Geometry check sheet. Reference: the model listing, model coordinates, mm. Face numbers are marked on the shaded views. A direction names the side the tool comes from. Coordinates: 2 decimals unless noted, no trailing zeros. Loops run counter-clockwise (first coordinate to the right, second up) from the corner with the lowest first, then second, coordinate; pieces in that order, holes last. Notation, with made-up numbers: M -4,40 L 6,40 A16 cw 6,66 Z; hole C -33,-36.75 d8. An arc over 180 degrees is marked long. One line per question, with ' | ' between items. Start each with the question number.
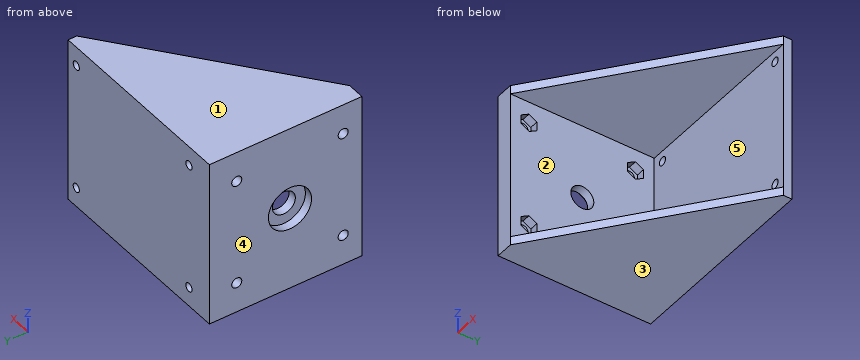
Autodesk Inventor part; units mm, degrees
ref_plane "YZ Plane" through (0, 0, 0) normal (1, 0, 0) x (0, 1, 0)
ref_plane "XZ Plane" through (0, 0, 0) normal (0, 1, 0) x (-1, 0, 0)
ref_plane "XY Plane" through (0, 0, 0) normal (0, 0, 1) x (1, 0, 0)
sketch "Skizze1" plane through (0, 0, 0) normal (0, 1, 0) x (-1, 0, 0)
  line L0 (-31.5, -26) -> (31.5, -26)
  line L1 (31.5, -26) -> (31.5, 26)
  line L2 (31.5, 26) -> (-31.5, 26)
  line L3 (-31.5, 26) -> (-31.5, -26)
  line L4 (-31.5, -26) -> (31.5, 26) construction
  line L5 (31.5, -26) -> (-31.5, 26) construction
  circle A0 centre (27.5, 22.25) radius 1.5
  circle A1 centre (-27.5, 22.25) radius 1.5
  circle A2 centre (-27.5, -22.25) radius 1.5
  circle A3 centre (27.5, -22.25) radius 1.5
  line L6 (31.5, 0) -> (-31.5, 0) construction
  line L7 (0, 26) -> (0, -26) construction
  line L8 (31.5, -26) -> (31.5, 26)
  line L9 (31.5, 26) -> (37.5, 26)
  line L10 (37.5, 26) -> (37.5, -26)
  line L11 (37.5, -26) -> (31.5, -26)
  point P0 (0, 0)
  dimension "d0" = 63
  dimension "d1" = 52
  dimension "d4" = 3
  dimension "d9" = 44.5
  dimension "d10" = 55
  dimension "d11" = 6
extrude "Extrusion1" add sketch "Skizze1" along normal blind 3
extrude "Extrusion2" add sketch "Skizze1" against normal blind 50 contours L1 L9 L10 L11
sketch "Skizze2" plane through (-31.5, -50, 26) normal (1, 0, 0) x (0, 0, -1)
  line L0 (52, 0) -> (0, 0)
  line L1 (26, 50) -> (26, 0) construction
  line L2 (7.5, 6.5) -> (44.5, 6.5)
  line L3 (44.5, 6.5) -> (44.5, 43.5)
  line L4 (44.5, 43.5) -> (7.5, 43.5)
  line L5 (7.5, 43.5) -> (7.5, 6.5)
  line L6 (7.5, 6.5) -> (44.5, 43.5) construction
  line L7 (44.5, 6.5) -> (7.5, 43.5) construction
  line L8 (42.9123, 3.75) -> (41.3246, 6.5)
  line L9 (41.3246, 6.5) -> (42.9123, 9.25)
  line L10 (42.9123, 9.25) -> (46.0877, 9.25)
  line L11 (46.0877, 9.25) -> (47.6754, 6.5)
  line L12 (47.6754, 6.5) -> (46.0877, 3.75)
  line L13 (46.0877, 3.75) -> (42.9123, 3.75)
  line L14 (5.9123, 3.75) -> (4.3246, 6.5)
  line L15 (4.3246, 6.5) -> (5.9123, 9.25)
  line L16 (5.9123, 9.25) -> (9.0877, 9.25)
  line L17 (9.0877, 9.25) -> (10.6754, 6.5)
  line L18 (10.6754, 6.5) -> (9.0877, 3.75)
  line L19 (9.0877, 3.75) -> (5.9123, 3.75)
  line L20 (41.3246, 43.5) -> (42.9123, 46.25)
  line L21 (42.9123, 46.25) -> (46.0877, 46.25)
  line L22 (46.0877, 46.25) -> (47.6754, 43.5)
  line L23 (47.6754, 43.5) -> (46.0877, 40.75)
  line L24 (46.0877, 40.75) -> (42.9123, 40.75)
  line L25 (42.9123, 40.75) -> (41.3246, 43.5)
  line L26 (4.3246, 43.5) -> (5.9123, 46.25)
  line L27 (5.9123, 46.25) -> (9.0877, 46.25)
  line L28 (9.0877, 46.25) -> (10.6754, 43.5)
  line L29 (10.6754, 43.5) -> (9.0877, 40.75)
  line L30 (9.0877, 40.75) -> (5.9123, 40.75)
  line L31 (5.9123, 40.75) -> (4.3246, 43.5)
  circle A0 centre (44.5, 6.5) radius 1.75
  circle A1 centre (7.5, 6.5) radius 1.75
  circle A2 centre (44.5, 43.5) radius 1.75
  circle A3 centre (7.5, 43.5) radius 1.75
  circle A4 centre (26, 25) radius 4
  point P0 (26, 25)
  dimension "d30" = 37
  dimension "d31" = 37
  dimension "d39" = 5.5
  dimension "d42" = 3.5
  dimension "d45" = 8
extrude "Extrusion4" cut sketch "Skizze2" against normal through all contours L5 A1 L2 | L2 A1 L5 | A0 L3 L2 | L2 L3 A0 | A3 L4 L5 | L5 L4 A3 | A2 L4 L3 | L3 L4 A2 | A4
extrude "Extrusion3" cut sketch "Skizze2" against normal blind 3 contours L5 A1 L2 | L2 A1 L5 | A1 L5 L16 L17 L2 | L2 L18 L19 L14 L15 L16 L5 A1 | L9 L10 L3 A0 L2 | L2 A0 L3 L10 L11 L12 L13 L8 | L30 L31 L26 L27 L28 L4 A3 L5 | L5 A3 L4 L29 L30 | A0 L3 L2 | L2 L3 A0 | A3 L4 L5 | L5 L4 A3 | L24 L25 L4 A2 L3 | L3 A2 L4 L20 L21 L22 L23 L24 | A2 L4 L3 | L3 L4 A2
sketch "Skizze3" plane through (31.5, 3, -26) normal (0, 0, -1) x (-1, 0, 0)
  line L0 (0, -3) -> (63, -3)
  line L1 (63, -3) -> (63, -53)
  line L2 (69, -53) -> (63, -53)
  line L3 (69, -53) -> (69, 0)
  line L4 (0, 0) -> (69, 0)
  line L5 (0, -3) -> (0, 0)
  line L6 (63, -53) -> (0, -3)
  point P0 (31.5, -3)
extrude "Extrusion5" add sketch "Skizze3" along normal blind 3
sketch "Skizze4" plane through (-37.5, 3, 26) normal (0, 0, 1) x (1, 0, 0)
  line L0 (6, -3) -> (69, -3)
  line L1 (69, -3) -> (69, 0)
  line L2 (0, 0) -> (69, 0)
  line L3 (0, -53) -> (0, 0)
  line L4 (6, -53) -> (0, -53)
  line L5 (6, -3) -> (6, -53)
  line L6 (6, -53) -> (69, -3)
  point P0 (37.5, -3)
extrude "Extrusion6" add sketch "Skizze4" along normal blind 3
sketch "Skizze5" plane through (-37.5, -50, -29) normal (-1, 0, 0) x (0, 0, 1)
  circle A0 centre (29, 25) radius 4
  circle A1 centre (29, 25) radius 7.5
  point P0 (29, 50)
  dimension "d51" = 15
extrude "Extrusion7" cut sketch "Skizze5" against normal blind 3
equation "\"d31\" = d30"
properties part number "Sanftanlauf_Halter"
1. Sectioned sample at B-B (y = -25). Record the cut outline in (x, z).
2. Sectioned sample at D-D (y = -36.5). Record the cut outline in (x, z).
3. Sectioned sample at C-C (z = 0). Record the cut outline in (x, y), and give its area (3 significant figures).
4. Tool access check on the marked faces 4 and 5. Record the directions out of +Z, -Z, +X, -X, +Y, -Y that give a thin tool (end or side, any length) a straight path to the whole face; none if there is none.
5. Depth check by flat-ended pin: pin 1 Ø10 at (x, y) = (-17, -41.5) entering from -Z; pin 2 Ø8 at (y, z) = (-38.5, 0.5) entering from +X; pin 3 Ø3 at (x, z) = (6, -17) entering from -Y. Enter the tip coordinate at first touch or a pass-through.
6. Thickness scan on line 1 (Y direction, x = -35.2, z = -18.5); line 2 (Z direction, x = -27.5, y = 1.3); line 3 (Z direction, x = -27, y = -7). Record the ranges inside material, lowest first.
7. Draft check along Z on the marked faces 1, 2 and 3. Enter one of: +Z half, -Z half, draft (parallel to the pull), parting line (faces both ways), or undercut.
8. Sectioned sample at A-A (z = -18.5). Record the cut outline in (x, y).
Result:
1) outline: M -37.5,-29 L 0,-29 L 0,-26 L -31.5,-26 L -31.5,-4 L -34.5,-4 L -34.5,-7.5 L -37.5,-7.5 Z; M -37.5,7.5 L -34.5,7.5 L -34.5,4 L -31.5,4 L -31.5,26 L 0,26 L 0,29 L -37.5,29 Z
2) outline: M -37.5,-29 L -14.49,-29 L -14.49,-26 L -31.5,-26 L -31.5,26 L -14.49,26 L -14.49,29 L -37.5,29 Z
3) outline: M -37.5,-50 L -31.5,-50 L -31.5,-29 L -34.5,-29 L -34.5,-32.5 L -37.5,-32.5 Z; M -37.5,-17.5 L -34.5,-17.5 L -34.5,-21 L -31.5,-21 L -31.5,0 L 31.5,0 L 31.5,3 L -37.5,3 Z | area: 438 mm2
4) face 4: +Z, -Z, -X, +Y, -Y | face 5: +X, -Y
5) pin 1: stops at z = -29 | pin 2: stops at x = -31.5 | pin 3: stops at y = 0
6) line 1: y = -50 to -45.25, -41.75 to -8.25, -4.75 to 3 | line 2: z = -29 to -23.75, -20.75 to 20.75, 23.75 to 29 | line 3: z = -29 to -26, 26 to 29
7) face 1: +Z half | face 2: undercut | face 3: -Z half
8) outline: M -37.5,-50 L -31.5,-50 L -31.5,-46.25 L -34.5,-46.25 L -34.5,-45.25 L -37.5,-45.25 Z; M -37.5,-41.75 L -34.5,-41.75 L -34.5,-40.75 L -31.5,-40.75 L -31.5,-9.25 L -34.5,-9.25 L -34.5,-8.25 L -37.5,-8.25 Z; M -37.5,-4.75 L -34.5,-4.75 L -34.5,-3.75 L -31.5,-3.75 L -31.5,0 L 31.5,0 L 31.5,3 L -37.5,3 Z
